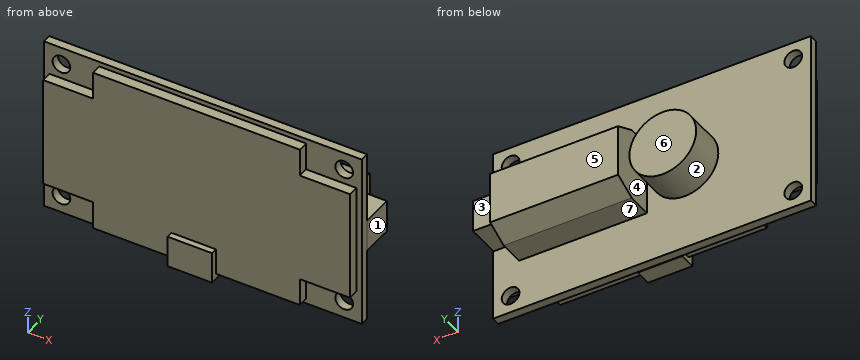
from build123d import *
from OCP.BRepFilletAPI import BRepFilletAPI_MakeChamfer

# Parameters (mm, degrees)
SKETCH1_W                = 57.15
SKETCH1_H                = 31.75
PCB_DEPTH                = 1.55
SKETCH2_R                = 1.59
MOUNT_HOLES_DEPTH        = 66.395622942
SKETCH4_R                = 6
SPEAKER_DEPTH            = 6.5
SKETCH5_W                = 23
SKETCH5_H                = 13.1
TERMINALS_DEPTH          = 8.5
CHAMFER1_SIZE            = 4
CHAMFER1_SIZE2           = 1.865230633
SKETCH7_W                = 4.5
SKETCH7_H                = 5.8
BATTERY_PORT_DEPTH       = 6
SKETCH11_W               = 8
SKETCH11_H               = 5.7
USB_PORT_DEPTH           = 3
SKETCH14_W               = 9
SKETCH14_H               = 20
SKETCH14_W_2             = 37.15
SKETCH14_H_2             = 30
SURFACE_COMPONENTS_DEPTH = 1.85


with BuildPart() as part:
    # Sketch1 → PCB (new body)
    with BuildSketch(Plane(origin=(0, 0, 0), x_dir=(1, 0, 0), z_dir=(0, 1, 0))):
        with Locations((28.575, -15.875)):
            Rectangle(SKETCH1_W, SKETCH1_H)
    extrude(amount=PCB_DEPTH)

    # Sketch2 → Mount Holes (cut, through all)
    with BuildSketch(Plane(origin=(0, 1.55, 0), x_dir=(1, 0, 0), z_dir=(0, 1, 0))):
        with Locations(Location((3.175, -3.175, 0), (0, 0, 270))):
            Circle(SKETCH2_R)
        with Locations(Location((3.175, -28.575, 0), (0, 0, 270))):
            Circle(SKETCH2_R)
        with Locations(Location((53.975, -28.575, 0), (0, 0, 270))):
            Circle(SKETCH2_R)
        with Locations(Location((53.975, -3.175, 0), (0, 0, 270))):
            Circle(SKETCH2_R)
    extrude(amount=-MOUNT_HOLES_DEPTH, mode=Mode.SUBTRACT)

    # Sketch4 → Speaker (add)
    with BuildSketch(Plane(origin=(0, 1.55, 0), x_dir=(1, 0, 0), z_dir=(0, 1, 0))):
        with Locations(Location((22.65, -15.875, 0), (0, 0, 90))):
            Circle(SKETCH4_R)
    extrude(amount=SPEAKER_DEPTH)

    # Sketch5 → Terminals (add)
    with BuildSketch(Plane(origin=(0, 1.55, 0), x_dir=(1, 0, 0), z_dir=(0, 1, 0))):
        with Locations((40.95, -15.875)):
            Rectangle(SKETCH5_W, SKETCH5_H)
    extrude(amount=TERMINALS_DEPTH)

    # Chamfer1: one chamfer whose edges measure the first distance from different faces: ONE call of the kernel's chamfer builder (chamfer() names one face for all edges)
    chamfer1_edges_1 = [part.edges().sort_by_distance(p)[0] for p in [
        (40.95, 10.05, 22.425),
    ]]
    chamfer1_side_1 = [part.faces().sort_by_distance(p)[0] for p in [
        (40.95, 5.8, 22.425),
    ]]
    chamfer1_edges_2 = [part.edges().sort_by_distance(p)[0] for p in [
        (40.95, 10.05, 9.325),
    ]]
    chamfer1_side_2 = [part.faces().sort_by_distance(p)[0] for p in [
        (40.95, 5.8, 9.325),
    ]]
    chamfer1 = BRepFilletAPI_MakeChamfer(part.part.solid().wrapped)
    for e in chamfer1_edges_1:
        chamfer1.Add(CHAMFER1_SIZE, CHAMFER1_SIZE2, e.wrapped, chamfer1_side_1[0].wrapped)  # the first distance lies on this face
    for e in chamfer1_edges_2:
        chamfer1.Add(CHAMFER1_SIZE, CHAMFER1_SIZE2, e.wrapped, chamfer1_side_2[0].wrapped)  # the first distance lies on this face
    add(Compound.cast(chamfer1.Shape()), mode=Mode.REPLACE)

    # Sketch7 → Battery Port (add)
    with BuildSketch(Plane(origin=(0, 1.55, 0), x_dir=(1, 0, 0), z_dir=(0, 1, 0))):
        with Locations((54.8, -15.875)):
            Rectangle(SKETCH7_W, SKETCH7_H)
    extrude(amount=BATTERY_PORT_DEPTH)



with BuildPart() as body_2:
    # Sketch11 → USB Port (new body)
    with BuildSketch(Plane(origin=(0, 0, 0), x_dir=(-1, 0, 0), z_dir=(0, -1, 0))):
        with Locations((-28.05, -2.75)):
            Rectangle(SKETCH11_W, SKETCH11_H)
    extrude(amount=USB_PORT_DEPTH)


with BuildPart() as part_1:
    add(part.part)

    add(body_2.part)  # Surface Components merges body 2
    # Sketch14 → Surface Components (add)
    with BuildSketch(Plane.XZ):
        with Locations((5.5, 15.875)):
            Rectangle(SKETCH14_W, SKETCH14_H)
        with Locations((28.575, 15.875)):
            Rectangle(SKETCH14_W_2, SKETCH14_H_2)
        with Locations((51.65, 15.875)):
            Rectangle(SKETCH14_W, SKETCH14_H)
    extrude(amount=SURFACE_COMPONENTS_DEPTH)


solid = part_1.part
The model under review builds one solid part; all positions refer to its coordinate system, in mm. Face numbers are marked on the shaded views. A direction names the side the tool comes from. Round coordinates to 2 decimals unless told otherwise and drop trailing zeros. Order: outer loops, then holes, each group sorted by start corner. A loop starts at its lowest first (then second) coordinate and runs counter-clockwise, first axis right, second up. Notation, with made-up numbers: (78, 41) -> (136, 41) arc R18 cw to (136, 67) -> close; hole circle Ø11 at (40.5, 61.5). An arc over 180 degrees is marked (long way). Write item = value, one per line. Start each with the question number.
Item 1: Consider section B-B on x = 38. Write out the cut boundary in (y, z) (3 decimals).
Item 2: For line 1 along Z through (x, y) = (24.5, 1.25); line 2 along Y through (x, z) = (50, 4); line 3 along Z through (x, y) = (25.5, -2), list the stretches that pass through material, from the lowest coordinate up.
Item 3: Consider section C-C on x = 49. Write out the cut boundary in (y, z) (3 decimals), plus the area to 3 significant figures.
Item 4: Mouldability with a two-part tool opening along X and no side actions: class the marked faces 1, 2 and 3 as released by +X, released by -X, zero draft, split by the parting line, or undercut.
Item 5: Consider section A-A on y = 3.25. Write out the cut boundary in (x, z) (3 decimals).
Item 6: Clearance check with flat-ended pins moving along their axes: pin 1 Ø4.5 at (y, z) = (4.5, 17) entering from +X; pin 2 Ø0.9 at (x, y) = (38.5, -1) entering from -Z (3 decimals); pin 3 Ø2 at (x, y) = (22.5, 1) entering from -Z. State where each tip first meets the part, or that it passes through.
Item 7: Consider section D-D on y = 6.75. Write out the cut boundary in (x, z) (3 decimals).
Item 8: For the marked faces 4, 5, 6 and 7, list the 3-axis set-ups (+Z, -Z, +X, -X, +Y, -Y) from which the entire face can be reached by the end or side of a thin tool; tool diameter is ignored.
Conclusion:
q1.outline = (-1.85, 0.875) -> (0, 0.875) -> (0, 0) -> (1.55, 0) -> (1.55, 9.325) -> (6.05, 9.325) -> (10.05, 11.19) -> (10.05, 20.56) -> (6.05, 22.425) -> (1.55, 22.425) -> (1.55, 31.75) -> (0, 31.75) -> (0, 30.875) -> (-1.85, 30.875) -> close
q2.line_1 = 0 to 31.75
q2.line_2 = 0 to 1.55
q2.line_3 = -0.1 to 5.6
q3.outline = (-1.85, 5.875) -> (0, 5.875) -> (0, 0) -> (1.55, 0) -> (1.55, 9.325) -> (6.05, 9.325) -> (10.05, 11.19) -> (10.05, 20.56) -> (6.05, 22.425) -> (1.55, 22.425) -> (1.55, 31.75) -> (0, 31.75) -> (0, 25.875) -> (-1.85, 25.875) -> close
q3.area = 190 mm2
q4.face_1 = released by +X
q4.face_2 = undercut
q4.face_3 = zero draft
q5.outline = circle Ø12 at (22.65, 15.875); (29.45, 9.325) -> (52.45, 9.325) -> (52.45, 22.425) -> (29.45, 22.425) -> close; (52.55, 12.975) -> (57.05, 12.975) -> (57.05, 18.775) -> (52.55, 18.775) -> close
q6.pin_1 = 57.05
q6.pin_2 = 0.875
q6.pin_3 = 0
q7.outline = circle Ø12 at (22.65, 15.875); (29.45, 9.651) -> (52.45, 9.651) -> (52.45, 22.099) -> (29.45, 22.099) -> close; (52.55, 12.975) -> (57.05, 12.975) -> (57.05, 18.775) -> (52.55, 18.775) -> close
q8.face_4 = +Z, -Z, +Y
q8.face_5 = +Z, -Z, +X, -X, +Y
q8.face_6 = +Z, -Z, -X, +Y
q8.face_7 = -Z, +X, -X, +Y
